Input: part model. Units: mm. Frame: model coordinates. A direction names the side the tool comes from. Round coordinates to 2 decimals unless told otherwise and drop trailing zeros. Order: outer loops, then holes, each group sorted by start corner. A loop starts at its lowest first (then second) coordinate and runs counter-clockwise, first axis right, second up. Notation, with made-up numbers: (45, 73.25) -> (99, 73.25) arc R12 cw to (99, 85.25) -> close; hole circle Ø6 at (87.25, 53). An arc over 180 degrees is marked (long way). Use a Markdown table: item, result.
from build123d import *

# Parameters (mm, degrees)
SKETCH1_W           = 6.5
SKETCH1_H           = 6
BOSS_EXTRUDE1_DEPTH = 1.8
SKETCH2_W           = 1
SKETCH2_H           = 0.8
BOSS_EXTRUDE2_DEPTH = 1.8
SKETCH3_R           = 1
BOSS_EXTRUDE3_DEPTH = 1.4
FILLET1_R           = 0.125


with BuildPart() as part:
    # Sketch1 → Boss-Extrude1 (new body)
    with BuildSketch(Plane(origin=(0, 0, 0), x_dir=(1, 0, 0), z_dir=(0, 1, 0))):
        Rectangle(SKETCH1_W, SKETCH1_H)
    extrude(amount=BOSS_EXTRUDE1_DEPTH)

    # Sketch2 → Boss-Extrude2 (add)
    with BuildSketch(Plane.XZ):
        with Locations((-2.8, 2)):
            Rectangle(SKETCH2_W, SKETCH2_H)
        with Locations((-2.8, -2)):
            Rectangle(SKETCH2_W, SKETCH2_H)
        with Locations((2.8, -2)):
            Rectangle(SKETCH2_W, SKETCH2_H)
        with Locations((2.8, 2)):
            Rectangle(SKETCH2_W, SKETCH2_H)
    extrude(amount=-BOSS_EXTRUDE2_DEPTH)

    # Sketch3 → Boss-Extrude3 (add)
    with BuildSketch(Plane(origin=(0, 1.8, 0), x_dir=(1, 0, 0), z_dir=(0, 1, 0))):
        with Locations(Location((0, 0, 0), (0, 0, 270))):
            Circle(SKETCH3_R)
    extrude(amount=BOSS_EXTRUDE3_DEPTH)

    # Fillet1
    fillet1_edges = [part.edges().sort_by_distance(p)[0] for p in [
        (-3.25, 0.9, -3),
        (3.25, 0.9, -3),
        (3.25, 0.9, 3),
        (-3.25, 0.9, 3),
    ]]
    fillet(fillet1_edges, radius=FILLET1_R)


solid = part.part
1) Cut plane D-D on z = 2. Return loops of the section in (x, y).
Results found:
| item | result |
|---|---|
| outline | (-3.3, 0) -> (3.3, 0) -> (3.3, 1.8) -> (-3.3, 1.8) -> close |
2) Cut plane C-C on y = 2.1. Return loops of the section in (x, z), and give its area (3 significant figures).
Results found:
| item | result |
|---|---|
| outline | circle Ø2 at (0, 0) |
| area | 3.14 mm² |
3) Line query: L1, parallel to Y at x = -0.25, z = -1.55; L2, parallel to X at y = 0.2, z = 0.5; L3, parallel to X at y = 2.15, z = 0.8. Output: solid intervals per line, ascending. Write a range as [from, to].
Results found:
| item | result |
|---|---|
| L1 | y = [0, 1.8] |
| L2 | x = [-3.25, 3.25] |
| L3 | x = [-0.6, 0.6] |
4) Pull-direction query (Z, two-part tool) for faces 1 (the flat face through (0, 0, 0)), 2 (the flat face through (3.25, 1, 0)), 3 (the cylindrical face through (-1, 2, 0)); classes: +Z half, -Z half, draft (parallel to the pull), parting line (faces both ways), or undercut.
Results found:
| item | result |
|---|---|
| face 1 | draft |
| face 2 | undercut |
| face 3 | parting line |
5) Cut plane A-A on z = 0. Return loops of the section in (x, y), and give its area (3 significant figures).
Results found:
| item | result |
|---|---|
| outline | (-3.25, 0) -> (3.25, 0) -> (3.25, 1.8) -> (1, 1.8) -> (1, 3.2) -> (-1, 3.2) -> (-1, 1.8) -> (-3.25, 1.8) -> close |
| area | 14.5 mm² |
6) Set-up query: faces 4 (the flat face through (-1, 1.8, 1)), 5 (the flat face through (-3.25, 1, 0)), 6 (the flat face through (0, 1, -3)). Return all of +Z, -Z, +X, -X, +Y, -Y with unobstructed straight access to the full face (end or side cutting, diameter ignored); none if empty.
Results found:
| item | result |
|---|---|
| face 4 | +Y |
| face 5 | -X, +Y, -Y |
| face 6 | -Z, +X, -X, +Y, -Y |
7) Pin query (flat end, axial travel): pin 1 Ø1.4 at (y, z) = (1, -0.5) entering from -X. Return the tip coordinate at first contact, or that it passes through.
Results found:
| item | result |
|---|---|
| pin 1 | stops at x = -3.25 |
8) Cut plane B-B on x = 0. Return loops of the section in (y, z).
Results found:
| item | result |
|---|---|
| outline | (0, -3) -> (1.8, -3) -> (1.8, -1) -> (3.2, -1) -> (3.2, 1) -> (1.8, 1) -> (1.8, 3) -> (0, 3) -> close |
